from build123d import *

# Parameters (mm, degrees)
SKETCH1_W           = 43.599999922
SKETCH1_H           = 29.050000066
BOSS_EXTRUDE1_DEPTH = 25.4


with BuildPart() as part:
    # Sketch1 → Boss-Extrude1 (new body)
    with BuildSketch(Plane.XY):
        Polygon((-28.149999961, -20.875000033), (-28.149999961, 20.875000033), (28.149999961, 20.875000033), (28.149999961, -20.875000033), (28.149999961, -93.900000033), (-28.149999961, -93.900000033), align=None)
        Rectangle(SKETCH1_W, SKETCH1_H, mode=Mode.SUBTRACT)
        Polygon((-19.245298339, -27.225000033), (0, -52.187485168), (19.245298339, -27.225000033), align=None, mode=Mode.SUBTRACT)
        Polygon((21.799999961, -34.311404785), (4.009049455, -57.387500033), (21.799999961, -80.463595281), align=None, mode=Mode.SUBTRACT)
        Polygon((-4.009049455, -57.387500033), (-21.799999961, -80.463595281), (-21.799999961, -34.311404785), align=None, mode=Mode.SUBTRACT)
        Polygon((0, -62.587514898), (-19.245298339, -87.550000033), (19.245298339, -87.550000033), align=None, mode=Mode.SUBTRACT)
    extrude(amount=BOSS_EXTRUDE1_DEPTH)


solid = part.part
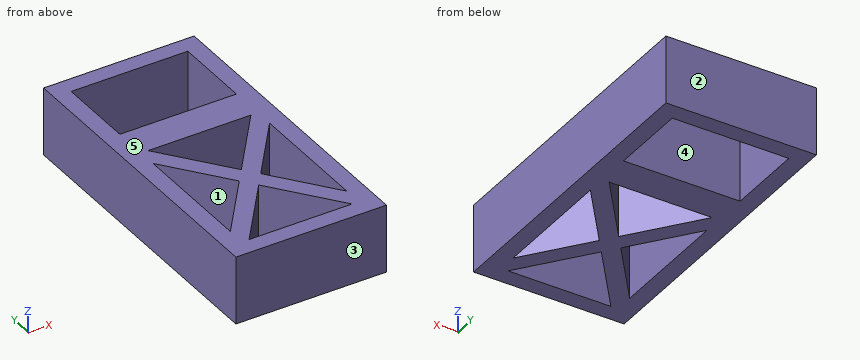
Work out the finished part from the listing and answer in its coordinate system (mm). Face numbers are marked on the shaded views. A direction names the side the tool comes from. Give positions to 0.01 mm unless a question says otherwise; leave off trailing zeros. Write each loop counter-clockwise with the first axis right and the second up, starting at its lowest first coordinate (ties: lowest second). Pieces come first, ordered by that corner, then holes. Notation, with made-up numbers: (41, 79.25) - (78, 79.25) arc R12 cw to (78, 91.25) - close; hole circle Ø5 at (-28, 16.25). An arc over 180 degrees is marked (long way). One line per item, written item: value. Start each with the question number.
1. Find section C-C (x = 2). Write down the section's boundary in (y, z) (3 decimals).
2. Given pin 1 (4 mm diameter, centred on x = 14.5, y = -72.5, fed in from -Z); pin 2 (8 mm diameter, centred on x = -17, y = -4.5, fed in from +Z), each flat-ended and moving along its own axis, determine where each tip first touches the part or whether it passes through.
3. For a pull along Y with two mould halves and no side action, classify the marked faces 1, 2 and 3 as +Y half, -Y half, draft (parallel to the pull), parting line (faces both ways), or undercut.
4. Find section A-A (z = 22.25). State how many separate pieces and enclosed holes the cut face has, then the cut area to 3 significant figures.
5. Find section D-D (y = -58.5). Write down the section's boundary in (x, z), then the cut area to 3 significant figures.
6. Consider probe 1 along Y at (x, z) = (0, 6.25) (3 decimals); probe 2 along X at (y, z) = (-7, 22); probe 3 along Y at (x, z) = (-14.5, 8.25) (3 decimals). Determine where each line is inside the solid, lowest interval first.
7. Find section B-B (y = 10.5). Write down the section's boundary in (x, z).
8. For the marked faces 4 and 5, determine the directions among +Z, -Z, +X, -X, +Y, -Y from which every point of the face is accessible in a straight line to the end or side of a thin tool.
Geometry results:
1. outline: (-93.9, 0) - (-87.55, 0) - (-87.55, 25.4) - (-93.9, 25.4) - close; (-65.182, 0) - (-49.593, 0) - (-49.593, 25.4) - (-65.182, 25.4) - close; (-27.225, 0) - (-14.525, 0) - (-14.525, 25.4) - (-27.225, 25.4) - close; (14.525, 0) - (20.875, 0) - (20.875, 25.4) - (14.525, 25.4) - close
2. pin 1: z = 0
2. pin 2: through
3. face 1: undercut
3. face 2: +Y half
3. face 3: -Y half
4. separate pieces: 1
4. enclosed holes: 5
4. area: 3,410 mm2
5. outline: (-28.15, 0) - (-21.8, 0) - (-21.8, 25.4) - (-28.15, 25.4) - close; (-4.87, 0) - (4.87, 0) - (4.87, 25.4) - (-4.87, 25.4) - close; (21.8, 0) - (28.15, 0) - (28.15, 25.4) - (21.8, 25.4) - close
5. area: 570 mm2
6. probe 1: -93.9 to -87.55, -62.588 to -52.187, -27.225 to -14.525, 14.525 to 20.875
6. probe 2: -28.15 to -21.8, 21.8 to 28.15
6. probe 3: -93.9 to -87.55, -81.395 to -70.995, -43.78 to -33.38, -27.225 to -14.525, 14.525 to 20.875
7. outline: (-28.15, 0) - (-21.8, 0) - (-21.8, 25.4) - (-28.15, 25.4) - close; (21.8, 0) - (28.15, 0) - (28.15, 25.4) - (21.8, 25.4) - close
8. face 4: +Z, -Z
8. face 5: +Z, +X, -X, +Y, -Y
